Work out the finished part from the listing and answer in its coordinate system (mm). A direction names the side the tool comes from. Round coordinates to 2 decimals unless told otherwise and drop trailing zeros. Order: outer loops, then holes, each group sorted by start corner. A loop starts at its lowest first (then second) coordinate and runs counter-clockwise, first axis right, second up. Notation, with made-up numbers: (-40, 14.5) - (-2, 14.5) arc R6 ccw to (-2, 19.5) - close; hole circle Ø9 at (5, 71.5). An arc over 180 degrees is marked (long way). Use CSV: the item, a comma, the result in double quotes.
from build123d import *

# Parameters (mm, degrees)
SKETCH1_W           = 79.375
SKETCH1_H           = 62.23
BOSS_EXTRUDE1_DEPTH = 24.13
SHELL1_T            = -3.81
RISER_BASE_SKETCH_R = 2.54
BOSS_EXTRUDE3_DEPTH = 2.54
SKETCH9_R           = 1.524
BOSS_EXTRUDE4_DEPTH = 2.54
SKETCH10_W          = 12.954
SKETCH10_H          = 10.922
CUT_EXTRUDE1_DEPTH  = 3.81
SKETCH12_W          = 9.254
SKETCH12_H          = 11.254
CUT_EXTRUDE2_DEPTH  = 3.81
SKETCH13_W          = 31.115
SKETCH13_H          = 24.13
CUT_EXTRUDE3_DEPTH  = 1.905
CHAMFER1_SIZE       = 0.889


with BuildPart() as part:
    # Sketch1 → Boss-Extrude1 (new body)
    with BuildSketch(Plane(origin=(0, 0, 0), x_dir=(1, 0, 0), z_dir=(0, 1, 0))):
        Rectangle(SKETCH1_W, SKETCH1_H)
    extrude(amount=-BOSS_EXTRUDE1_DEPTH)

    # Shell1
    shell1_openings = [part.faces().sort_by_distance(p)[0] for p in [
        (0, 0, 0),
    ]]
    offset(amount=SHELL1_T, openings=shell1_openings, kind=Kind.INTERSECTION)

    # riser base sketch → Boss-Extrude3 (add)
    with BuildSketch(Plane(origin=(0, -20.32, 0), x_dir=(1, 0, 0), z_dir=(0, 1, 0))):
        with Locations(Location((32.7025, 8.89, 0), (0, 0, 90))):
            Circle(RISER_BASE_SKETCH_R)
        with Locations(Location((-18.0975, 24.13, 0), (0, 0, 90))):
            Circle(RISER_BASE_SKETCH_R)
        with Locations(Location((-19.3675, -24.13, 0), (0, 0, 90))):
            Circle(RISER_BASE_SKETCH_R)
        with Locations(Location((32.7025, -19.05, 0), (0, 0, 90))):
            Circle(RISER_BASE_SKETCH_R)
    extrude(amount=BOSS_EXTRUDE3_DEPTH)

    # Sketch9 → Boss-Extrude4 (add)
    with BuildSketch(Plane(origin=(0, -17.78, 0), x_dir=(-1, 0, 0), z_dir=(0, 1, 0))):
        with Locations(Location((19.3675, 24.13, 0), (0, 0, 270))):
            Circle(SKETCH9_R)
        with Locations(Location((-32.7025, 19.05, 0), (0, 0, 270))):
            Circle(SKETCH9_R)
        with Locations(Location((-32.7025, -8.89, 0), (0, 0, 270))):
            Circle(SKETCH9_R)
        with Locations(Location((18.0975, -24.13, 0), (0, 0, 270))):
            Circle(SKETCH9_R)
    extrude(amount=BOSS_EXTRUDE4_DEPTH)

    # Sketch10 → Cut-Extrude1 (cut)
    with BuildSketch(Plane.ZY.offset(39.6875)):
        with Locations((-10.795, -11.176)):
            Rectangle(SKETCH10_W, SKETCH10_H)
    extrude(amount=-CUT_EXTRUDE1_DEPTH, mode=Mode.SUBTRACT)

    # Sketch12 → Cut-Extrude2 (cut)
    with BuildSketch(Plane.ZY.offset(39.6875)):
        with Locations((18.36, -11.01)):
            Rectangle(SKETCH12_W, SKETCH12_H)
    extrude(amount=-CUT_EXTRUDE2_DEPTH, mode=Mode.SUBTRACT)

    # Sketch13 → Cut-Extrude3 (cut)
    with BuildSketch(Plane.ZY.offset(39.6875)):
        with Locations((15.5575, -12.065)):
            Rectangle(SKETCH13_W, SKETCH13_H)
    extrude(amount=-CUT_EXTRUDE3_DEPTH, mode=Mode.SUBTRACT)

    # Chamfer1
    chamfer1_edges = [part.edges().sort_by_distance(p)[0] for p in [
        (-39.6875, -24.13, -15.5575),
        (35.8775, 0, 0),
        (0, 0, -27.305),
        (-35.8775, 0, 0),
        (0, 0, 27.305),
        (39.6875, -24.13, 0),
        (-39.6875, 0, -15.5575),
        (0, 0, -31.115),
        (39.6875, 0, 0),
        (-39.6875, -11.176, -17.272),
        (-39.6875, -16.637, -10.795),
        (-39.6875, -11.176, -4.318),
        (-39.6875, -5.715, -10.795),
        (0, -24.13, -31.115),
        (39.6875, -12.065, 31.115),
        (-39.6875, -12.065, -31.115),
        (39.6875, -12.065, -31.115),
        (-37.7825, -16.637, 18.36),
        (0.9525, -24.13, 31.115),
        (0.9525, 0, 31.115),
        (-39.6875, -12.065, 0),
        (-37.7825, -12.065, 31.115),
        (-37.7825, -24.13, 15.5575),
        (-37.7825, -12.065, 0),
        (-38.735, -24.13, 0),
        (-37.7825, 0, 15.5575),
        (-38.735, 0, 0),
        (-37.7825, -11.01, 13.733),
        (-37.7825, -5.383, 18.36),
        (-37.7825, -11.01, 22.987),
    ]]
    chamfer(chamfer1_edges, length=CHAMFER1_SIZE)


solid = part.part
(1) Find section B-B (z = -8.89). Determine the outline of the cut face in (x, y) (1 decimal), and give its area (3 significant figures).
Findings below:
outline,"(-39.7, -23.2) - (-38.8, -24.1) - (38.8, -24.1) - (39.7, -23.2) - (39.7, -0.9) - (38.8, 0) - (36.8, 0) - (35.9, -0.9) - (35.9, -20.3) - (35.2, -20.3) - (35.2, -17.8) - (34.2, -17.8) - (34.2, -15.2) - (31.2, -15.2) - (31.2, -17.8) - (30.2, -17.8) - (30.2, -20.3) - (-35.9, -20.3) - (-35.9, -16.6) - (-38.8, -16.6) - (-39.7, -17.5) - close; (-39.7, -4.8) - (-38.8, -5.7) - (-35.9, -5.7) - (-35.9, -0.9) - (-36.8, 0) - (-38.8, 0) - (-39.7, -0.9) - close"
area,"433 mm²"
(2) Each of these flat-tipped pins is pushed along its axis until it touches: pin 1 (2.5 mm diameter, centred on x = 33, z = 18.5, fed in from +Y); pin 2 (1.5 mm diameter, centred on x = 22.5, z = 11.5, fed in from +Y); pin 3 (0.9 mm diameter, centred on x = -37.5, y = -10, fed in from +Z). Where does it stop, or does it pass through?
Findings below:
pin 1,"stops at y = -15.24"
pin 2,"stops at y = -20.32"
pin 3,"stops at z = 30.96"
(3) Find the intervals of material crossed by L1, parallel to Z at x = -36, y = -12.75 (3 decimals); L2, parallel to Z at x = 34.5, y = -2.75 (3 decimals); L3, parallel to X at y = -11, z = 9.5, in increasing order. Write a range as from..to.
Findings below:
L1,"z = -31.115..-17.272, -4.318..13.733, 22.987..31.115"
L2,"z = -31.115..-27.305, 27.305..31.115"
L3,"x = -37.78..-35.88, 35.88..39.69"
(4) For faces 1 (the flat face through (-37, -5.715, -11)), 2 (the flat face through (0, -12, 31.115)), 3 (the flat face through (33, -15.24, -9)), 4 (the cylindrical face through (-21.084, -19.068, 26.002)), determine the directions among +Z, -Z, +X, -X, +Y, -Y from which every point of the face is accessible in a straight line to the end or side of a thin tool.
Findings below:
face 1,"-X"
face 2,"+Z, +X, -X, +Y, -Y"
face 3,"-X, +Y"
face 4,"+Y"
(5) Find section C-C (x = -3.5). Determine the outline of the cut face in (y, z) (3 decimals), and give its area (3 significant figures).
Findings below:
outline,"(-24.13, -30.226) - (-23.241, -31.115) - (-0.889, -31.115) - (0, -30.226) - (0, -28.194) - (-0.889, -27.305) - (-20.32, -27.305) - (-20.32, 27.305) - (-0.889, 27.305) - (0, 28.194) - (0, 30.226) - (-0.889, 31.115) - (-23.241, 31.115) - (-24.13, 30.226) - close"
area,"390 mm²"
(6) The mould has two halves that part along Z. Classify faces 5 (the flat face through (6, 0, -29)), 6 (the flat face through (-37.97, -23.78, 0.16)), 7 (the flat face through (-37, -11, -17.272)): released by +Z, released by -Z, zero draft, split by the parting line, or undercut.
Findings below:
face 5,"zero draft"
face 6,"released by +Z"
face 7,"undercut"
(7) Find section D-D (z = -19). Determine the outline of the cut face in (x, y), and give its area (3 significant figures).
Findings below:
outline,"(-39.69, -23.24) - (-38.8, -24.13) - (38.8, -24.13) - (39.69, -23.24) - (39.69, -0.89) - (38.8, 0) - (36.77, 0) - (35.88, -0.89) - (35.88, -20.32) - (-35.88, -20.32) - (-35.88, -0.89) - (-36.77, 0) - (-38.8, 0) - (-39.69, -0.89) - close"
area,"455 mm²"
